```python
from build123d import *

# Parameters (mm, degrees)
BOSS_EXTRUDE1_DEPTH       = 1.5875
F_4_CLEARANCE_HOLE1_D     = 3.4
F_4_CLEARANCE_HOLE1_DEPTH = 1.5875
HOLE1_D                   = 18
HOLE1_DEPTH               = 1.5875
CHAMFER1_SIZE             = 0.5
FILLET1_R                 = 10


with BuildPart() as part:
    # Sketch1 → Boss-Extrude1 (new body)
    with BuildSketch(Plane.XY.offset(1.5875)):
        with BuildLine():
            Line((-122.373252992, 49.591627472), (-33.137949262, 9.81285715))
            Line((-33.137949262, 9.81285715), (-12.780339067, 55.480873389))
            Line((-12.780339067, 55.480873389), (-102.015642796, 95.25964371))
            ThreePointArc((-102.015642796, 95.25964371), (-106.983028684, 96.085831021), (-111.723245825, 94.386463641))
            Line((-111.723245825, 94.386463641), (-171.498000771, 121.032489918))
            ThreePointArc((-171.498000771, 121.032489918), (-198.238379477, 110.781775471), (-187.98766503, 84.041396765))
            Line((-187.98766503, 84.041396765), (-128.212910083, 57.395370488))
            ThreePointArc((-128.212910083, 57.395370488), (-126.308202352, 52.73386896), (-122.373252992, 49.591627472))
        make_face()
    extrude(amount=-BOSS_EXTRUDE1_DEPTH)

    # #4 Clearance Hole1
    with Locations(Plane.XY.offset(1.5875)):
        with Locations((-99.517086056, 91.408706914), (-62.982673065, 75.122618757), (-26.448260075, 58.836530601), (-20.722062659, 44.787930558), (-30.493715553, 22.867282764), (-44.77010925, 17.735315986), (-81.304522241, 34.021404143), (-117.838935231, 50.307492299), (-131.618242769, 99.970559768), (-145.664993804, 68.459628564), (-173.979163871, 81.081346885), (-159.932412836, 112.592278089), (-192.145991763, 114.525444092), (-196.950263565, 103.748070885)):
            Hole(F_4_CLEARANCE_HOLE1_D / 2, depth=F_4_CLEARANCE_HOLE1_DEPTH)

    # Hole1
    with Locations(Plane(origin=(0, 0, 0), x_dir=(-1, 0, 0), z_dir=(0, 0, -1))):
        with Locations((179.7428329, 102.536943342)):
            Hole(HOLE1_D / 2, depth=HOLE1_DEPTH)

    # Chamfer1
    chamfer1_edges = [part.edges().sort_by_distance(p)[0] for p in [
        (-24.748260075, 58.836530601, 1.5875),
        (-61.282673065, 75.122618757, 1.5875),
        (-97.817086056, 91.408706914, 1.5875),
        (-195.250263565, 103.748070885, 1.5875),
        (-190.445991763, 114.525444092, 1.5875),
        (-158.232412836, 112.592278089, 1.5875),
        (-172.279163871, 81.081346885, 1.5875),
        (-143.964993804, 68.459628564, 1.5875),
        (-129.918242769, 99.970559768, 1.5875),
        (-116.138935231, 50.307492299, 1.5875),
        (-79.604522241, 34.021404143, 1.5875),
        (-43.07010925, 17.735315986, 1.5875),
        (-28.793715553, 22.867282764, 1.5875),
        (-19.022062659, 44.787930558, 1.5875),
    ]]
    chamfer(chamfer1_edges, length=CHAMFER1_SIZE)

    # Fillet1
    fillet1_edges = [part.edges().sort_by_distance(p)[0] for p in [
        (-12.780339067, 55.480873389, 0.79375),
        (-33.137949262, 9.81285715, 0.79375),
    ]]
    fillet(fillet1_edges, radius=FILLET1_R)


solid = part.part
```
Geometry check sheet. Reference: the model listing, model coordinates, mm. Give positions to 0.01 mm unless a question says otherwise; leave off trailing zeros. Order: outer loops, then holes, each group sorted by start corner. A loop starts at its lowest first (then second) coordinate and runs counter-clockwise, first axis right, second up. Notation, with made-up numbers: (-12.5, -23.5) - (30.5, -23.5) arc R22 ccw to (30.5, -8.5) - close; hole circle Ø3 at (38, -12). An arc over 180 degrees is marked (long way). Answer in a Markdown table with one row per item. Add a question column.
Q1. Mould release check, pull along X, two halves, no side actions. Record for faces 1 (the cylindrical face through (-126.35, 52.79, 0.8)), 2 (the cylindrical face through (-192.9, 113, 0.5)), 3 (the flat face through (-109, 69, 1.588)): pulls with the +X half, pulls with the -X half, needs draft (parallel to the pull), parting line crosses it, or undercut.
Q2. Cross-section at B-B, the plane x = -164. Enter the section's corners in (y, z).
Q3. Gauge pin test, flat end, axial feed: pin 1 (2 mm diameter, centred on x = -30.49, y = 22.87, fed in from +Z). Record the tip position at first contact, or that the pin passes through.
Q4. Material ranges on probe 1 along Y at (x, z) = (-188, 1.15); probe 2 along X at (y, z) = (50, 0.2); probe 3 along X at (y, z) = (80.5, 0.45), recorded low to high. Write a range as from..to.
Q5. Cross-section at C-C, the plane y = 54.5. Enter the section's corners in (x, z), then the cut area to 3 significant figures.
Q6. Cross-section at A-A, the plane z = 0.5. Count the separate pieces of the cut face and the enclosed holes in it, then the cut area to 3 significant figures.
Check values:
| question | item | result |
|---|---|---|
| 1 | face 1 | pulls with the -X half |
| 1 | face 2 | undercut |
| 1 | face 3 | needs draft |
| 2 | outline | (73.35, 0) - (117.69, 0) - (117.69, 1.59) - (73.35, 1.59) - close |
| 3 | pin 1 | passes through |
| 4 | probe 1 | y = 84.05..98.96, 106.12..121.03 |
| 4 | probe 2 | x = -123.19..-119.51, -116.17..-15.99 |
| 4 | probe 3 | x = -180.04..-175.58, -172.38..-68.91 |
| 5 | outline | (-127.37, 0) - (-16.86, 0) - (-16.86, 1.59) - (-127.37, 1.59) - close |
| 5 | area | 175 mm^2 |
| 6 | separate pieces | 1 |
| 6 | enclosed holes | 15 |
| 6 | area | 8,160 mm^2 |
